Verification items for the finished model (mm, model axes). Round coordinates to 2 decimals unless told otherwise and drop trailing zeros. Write each loop counter-clockwise with the first axis right and the second up, starting at its lowest first coordinate (ties: lowest second). Pieces come first, ordered by that corner, then holes. Notation, with made-up numbers: (44.25, -21) - (74.25, -21) arc R28 ccw to (74.25, -1) - close; hole circle Ø7 at (44, -12.5). An arc over 180 degrees is marked (long way). Answer as a JSON object with one key per item and string values. Group by question number.
1) Section check C-C (z = -0.5). Enter the section's corners in (x, y).
2) Section check D-D (y = -3.35). Enter the section's corners in (x, z).
3) Section check A-A (x = 0). Enter the section's corners in (y, z).
4) Go/stop test with flat-tipped pins: pin 1 Ø2.5 at (x, z) = (0, -22.39) entering from -Y; pin 2 Ø2.5 at (x, z) = (0, 22.39) entering from +Y; pin 3 Ø1.2 at (x, y) = (1, -4.5) entering from +Z. Record where each tip stops, or that it passes through.
5) Section check B-B (y = -0.9). Enter the section's corners in (x, z), then the cut area to 3 significant figures.
6) Thickness scan on line 1 (Z direction, x = 0, y = -3.05); line 2 (X direction, y = -0.25, z = 2); line 3 (Z direction, x = 0.7, y = -2.5) (3 decimals). Record the ranges inside material, lowest first.
```python
from build123d import *

# Parameters (mm, degrees)
F0_W     = 5.588
F0_H     = 33.6042
F0_R     = 0.9906
F1_DEPTH = 5.588
F2_W     = 1.4605
F2_H     = 2.5908
F2_H_2   = 2.794
F3_DEPTH = 5.589


with BuildPart() as f1:
    # F0 (on Front) → F1 (new body)
    with BuildSketch(Plane.XZ):
        Rectangle(F0_W, F0_H)
        with BuildLine():
            ThreePointArc((-0.9271, 14.986), (0, 15.9131), (0.9271, 14.986))
            Line((0.9271, 14.986), (0.9271, -14.986))
            ThreePointArc((0.9271, -14.986), (0, -15.9131), (-0.9271, -14.986))
            Line((-0.9271, -14.986), (-0.9271, 14.986))
        make_face(mode=Mode.SUBTRACT)
        with BuildLine():
            Line((-2.794, 16.8021), (2.794, 16.8021))
            Line((2.794, 16.8021), (2.794, 22.3901))
            ThreePointArc((2.794, 22.3901), (0, 25.1841), (-2.794, 22.3901))
            Line((-2.794, 22.3901), (-2.794, 16.8021))
        make_face()
        with Locations((0, 22.3901)):
            Circle(F0_R, mode=Mode.SUBTRACT)
        with BuildLine():
            Line((2.794, -22.3901), (2.794, -16.8021))
            Line((2.794, -16.8021), (-2.794, -16.8021))
            Line((-2.794, -16.8021), (-2.794, -22.3901))
            ThreePointArc((-2.794, -22.3901), (0, -25.1841), (2.794, -22.3901))
        make_face()
        with Locations((0, -22.3901)):
            Circle(F0_R, mode=Mode.SUBTRACT)
    extrude(amount=F1_DEPTH)

    # F2 (on face) → F3 (cut, through all)
    with BuildSketch(Plane(origin=(-2.794, 0, 0), x_dir=(0, -1, 0), z_dir=(-1, 0, 0))):
        with Locations((0.73025, 21.0947)):
            Rectangle(F2_W, F2_H)
        with Locations((0.73025, 23.7871)):
            Rectangle(F2_W, F2_H_2)
        with Locations((4.85775, 23.7871)):
            Rectangle(F2_W, F2_H_2)
        with Locations((4.85775, 21.0947)):
            Rectangle(F2_W, F2_H)
        with Locations((0.73025, -23.7871)):
            Rectangle(F2_W, F2_H_2)
        with Locations((0.73025, -21.0947)):
            Rectangle(F2_W, F2_H)
        with Locations((4.85775, -21.0947)):
            Rectangle(F2_W, F2_H)
        with Locations((4.85775, -23.7871)):
            Rectangle(F2_W, F2_H_2)
    extrude(amount=-F3_DEPTH, mode=Mode.SUBTRACT)


solid = f1.part
```
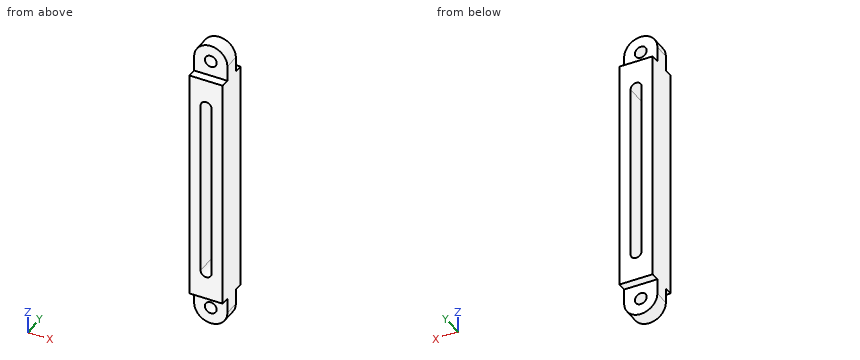
Returned:
{
 "1": {"outline": "(-2.79, -5.59) - (-0.93, -5.59) - (-0.93, 0) - (-2.79, 0) - close; (0.93, -5.59) - (2.79, -5.59) - (2.79, 0) - (0.93, 0) - close"},
 "2": {"outline": "(-2.79, -22.39) arc R2.79 ccw to (2.79, -22.39) - (2.79, 22.39) arc R2.79 ccw to (-2.79, 22.39) - close; hole circle Ø1.98 at (0, -22.39); hole circle Ø1.98 at (0, 22.39); hole (-0.93, -14.99) arc R0.93 ccw to (0.93, -14.99) - (0.93, 14.99) arc R0.93 ccw to (-0.93, 14.99) - close"},
 "3": {"outline": "(-5.59, -19.8) - (-4.13, -19.8) - (-4.13, -21.4) - (-1.46, -21.4) - (-1.46, -19.8) - (0, -19.8) - (0, -15.91) - (-5.59, -15.91) - close; (-5.59, 15.91) - (0, 15.91) - (0, 19.8) - (-1.46, 19.8) - (-1.46, 21.4) - (-4.13, 21.4) - (-4.13, 19.8) - (-5.59, 19.8) - close; (-4.13, -25.18) - (-1.46, -25.18) - (-1.46, -23.38) - (-4.13, -23.38) - close; (-4.13, 23.38) - (-1.46, 23.38) - (-1.46, 25.18) - (-4.13, 25.18) - close"},
 "4": {"pin 1": "y = -4.13", "pin 2": "y = -1.46", "pin 3": "z = 25.13"},
 "5": {"outline": "(-2.79, -19.8) - (2.79, -19.8) - (2.79, 19.8) - (-2.79, 19.8) - close; hole (-0.93, -14.99) arc R0.93 ccw to (0.93, -14.99) - (0.93, 14.99) arc R0.93 ccw to (-0.93, 14.99) - close", "area": "163 mm2"},
 "6": {"line 1": "-25.18 to -23.38, -21.4 to -15.91, 15.91 to 21.4, 23.38 to 25.18", "line 2": "-2.79 to -0.93, 0.93 to 2.79", "line 3": "-25.095 to -23.091, -21.689 to -15.594, 15.594 to 21.689, 23.091 to 25.095"}
}
